Read the model definition and answer for the solid it produces. Units are mm, in the model's axes. Face numbers are marked on the shaded views. A direction names the side the tool comes from. Coordinates: 2 decimals unless noted, no trailing zeros. Write each loop counter-clockwise with the first axis right and the second up, starting at its lowest first coordinate (ties: lowest second). Pieces come first, ordered by that corner, then holes.
Item 1: A tool of negligible diameter and unlimited length cuts with its end or side. For the marked faces 1 and 2, from which of +Z, -Z, +X, -X, +Y, -Y can it reach the whole face along a straight path? Write none if from no direction.
Item 2: Straight lines are drawn through the part: probe 1 along X at (y, z) = (0, 12); probe 2 along X at (y, z) = (0, 1.2); probe 3 along Y at (x, z) = (32, 3). For each, find the intervals that lie inside material, in ascending order.
Item 3: Each of these flat-tipped pins is pushed along its axis until it touches: P1, Ø6, axis at x = -32, y = 0, coming from the +Z side; P2, Ø5, axis at x = -9.5, y = -26, coming from the -Z side; P3, Ø10, axis at x = 31, y = 2, coming from the +Z side. Where does it stop, or does it pass through?
Item 4: Section D-D (z = 31) is taken. Give the vertices of the cut face in (x, y), then the cut area to 3 significant figures.
Item 5: Section A-A (x = -2) is taken. Give the vertices of the cut face in (y, z), then the cut area to 3 significant figures.
Item 6: Section B-B (x = -32) is taken. Give the vertices of the cut face in (y, z), then the cut area to 3 significant figures.
Item 7: Section C-C (y = -16.5) is taken. Give the vertices of the cut face in (x, z).
from build123d import *

# Parameters (mm, degrees)
SKETCH1_W                = 80
SKETCH1_H                = 20
BOSS_EXTRUDE1_DEPTH      = 5
BOSS_EXTRUDE2_DEPTH      = 90
BOSS_EXTRUDE2_DEPTH_BACK = 64
SKETCH4_W                = 114
SKETCH4_H                = 22
CUT_EXTRUDE2_DEPTH       = 109.466361883
CHAMFER2_SIZE            = 11.3
CHAMFER2_SIZE_2          = 15.980613255
CHAMFER4_SIZE            = 5
CHAMFER4_SIZE2           = 10.722534603
CUT_EXTRUDE1_DEPTH       = 109.942423601
CUT_EXTRUDE1_DEPTH_BACK  = 109.942423601
SKETCH2_R                = 2.3
SKETCH5_R                = 4.5
CUT_EXTRUDE3_DEPTH       = 107.728174912
SKETCH6_R                = 1.5
CUT_EXTRUDE4_DEPTH       = 5
FILLET2_R                = 5.6


with BuildPart() as part:
    # Sketch1 → Boss-Extrude1 (new body)
    with BuildSketch(Plane.XY):
        Rectangle(SKETCH1_W, SKETCH1_H)
    extrude(amount=BOSS_EXTRUDE1_DEPTH)

    # Sketch3 → Boss-Extrude2 (add, two sides: drawn at the far end of the back side and taken through both)
    with BuildSketch(Plane(origin=(0, 0, 0), x_dir=(0, 0, -1), z_dir=(1, 0, 0)).offset(-BOSS_EXTRUDE2_DEPTH_BACK)):
        Polygon((-5, 10), (-50.254833996, -35.254833996), (-46.012193309, -35.254833996), (-5, 5.757359313), align=None)
    extrude(amount=BOSS_EXTRUDE2_DEPTH + BOSS_EXTRUDE2_DEPTH_BACK)

    # Sketch4 → Cut-Extrude2 (cut, through all)
    with BuildSketch(Plane(origin=(0, 5.378679656, 5.378679656), x_dir=(1, 0, 0), z_dir=(0, -0.7071067811865509, -0.7071067811865441))):
        with Locations((13, 33.464466094)):
            Rectangle(SKETCH4_W, SKETCH4_H)
    extrude(amount=-CUT_EXTRUDE2_DEPTH, mode=Mode.SUBTRACT)

    # Chamfer1
    # the kernel refuses this chamfer: 5 mm, written as the material it adds along each edge
    with BuildSketch(Plane(origin=(40, -25.102836543, 5), x_dir=(-0.027495876610586317, 0, -0.9996219169112968), z_dir=(0, 1, 0))) as chamfer1_piece_1_section:
        with BuildLine():
            Line((5.143365976, 0), (-0.282735774, -5.135588968))
            Line((-0.282735774, -5.135588968), (-0.382697966, -5.13283938))
            ThreePointArc((-0.382697966, -5.13283938), (-0.170646135, -2.566989148), (-0.099962192, 0.002749588))
            Line((-0.099962192, 0.002749588), (0.002749588, 0.099962192))
            ThreePointArc((0.002749588, 0.099962192), (2.572488324, 0.029278248), (5.146115564, 0.099962192))
            Line((5.146115564, 0.099962192), (5.143365976, 0))
        make_face()
    chamfer1_piece_1 = extrude(amount=35.102836543, mode=Mode.PRIVATE)
    chamfer1_piece_1 = split(chamfer1_piece_1, bisect_by=Plane(origin=(41.544288895, -10, 3.190389103), z_dir=(0, 1, 0)), keep=Keep.TOP, mode=Mode.PRIVATE)
    chamfer1_piece_1 = split(chamfer1_piece_1, bisect_by=Plane(origin=(41.544288895, -1.222319508, 0), z_dir=(0, 0, 1)), keep=Keep.TOP, mode=Mode.PRIVATE)
    chamfer1_piece_1 = split(chamfer1_piece_1, bisect_by=Plane(origin=(41.544288895, -1.222319508, 5), z_dir=(0, 0, -1)), keep=Keep.TOP, mode=Mode.PRIVATE)
    chamfer1_piece_1 = split(chamfer1_piece_1, bisect_by=Plane(origin=(41.544288895, 3.172325351, 7.585033962), z_dir=(0, -0.7071067811865511, -0.707106781186544)), keep=Keep.TOP, mode=Mode.PRIVATE)
    add(chamfer1_piece_1)
    with BuildSketch(Plane(origin=(40, -25.102836543, 5), x_dir=(-0.027495876610586317, 0, -0.9996219169112968), z_dir=(0, 1, 0))) as chamfer1_piece_2_section:
        with BuildLine():
            Line((5.143365976, 0), (-0.282735774, -5.135588968))
            Line((-0.282735774, -5.135588968), (-0.382697966, -5.13283938))
            ThreePointArc((-0.382697966, -5.13283938), (-0.170646135, -2.566989148), (-0.099962192, 0.002749588))
            Line((-0.099962192, 0.002749588), (0.002749588, 0.099962192))
            ThreePointArc((0.002749588, 0.099962192), (2.572488324, 0.029278248), (5.146115564, 0.099962192))
            Line((5.146115564, 0.099962192), (5.143365976, 0))
        make_face()
    chamfer1_piece_2 = extrude(amount=35.102836543, mode=Mode.PRIVATE)
    chamfer1_piece_2 = split(chamfer1_piece_2, bisect_by=Plane(origin=(41.882166071, 8.451075781, 5), z_dir=(0, 0, -1)), keep=Keep.TOP, mode=Mode.PRIVATE)
    chamfer1_piece_2 = split(chamfer1_piece_2, bisect_by=Plane(origin=(41.882166071, 7.676613671, 3.080745642), z_dir=(0, 0.7071067811865511, 0.707106781186544)), keep=Keep.TOP, mode=Mode.PRIVATE)
    add(chamfer1_piece_2)
    with BuildSketch(Plane(origin=(40, -25.102836543, 5), x_dir=(-0.027495876610586317, 0, -0.9996219169112968), z_dir=(0, 1, 0))) as chamfer1_piece_3_section:
        with BuildLine():
            Line((5.143365976, 0), (-0.282735774, -5.135588968))
            Line((-0.282735774, -5.135588968), (-0.382697966, -5.13283938))
            ThreePointArc((-0.382697966, -5.13283938), (-0.170646135, -2.566989148), (-0.099962192, 0.002749588))
            Line((-0.099962192, 0.002749588), (0.002749588, 0.099962192))
            ThreePointArc((0.002749588, 0.099962192), (2.572488324, 0.029278248), (5.146115564, 0.099962192))
            Line((5.146115564, 0.099962192), (5.143365976, 0))
        make_face()
    chamfer1_piece_3 = extrude(amount=35.102836543, mode=Mode.PRIVATE)
    chamfer1_piece_3 = split(chamfer1_piece_3, bisect_by=Plane(origin=(43.003980886, 7.808289703, 5), z_dir=(0, 0, 1)), keep=Keep.TOP, mode=Mode.PRIVATE)
    chamfer1_piece_3 = split(chamfer1_piece_3, bisect_by=Plane(origin=(43.003980886, 6.747629531, 4.009729782), z_dir=(0, 0.7071067811865511, 0.707106781186544)), keep=Keep.TOP, mode=Mode.PRIVATE)
    chamfer1_piece_3 = split(chamfer1_piece_3, bisect_by=Plane(origin=(43.003980886, 8.868949875, 6.131050125), z_dir=(0, -0.7071067811865511, -0.7071067811865439)), keep=Keep.TOP, mode=Mode.PRIVATE)
    add(chamfer1_piece_3)
    with BuildSketch(Plane(origin=(-40, 10, 5), x_dir=(0.027495876610586317, 0, -0.9996219169112968), z_dir=(0, -1, 0))) as chamfer1_piece_4_section:
        with BuildLine():
            Line((5.143365976, 0), (-0.282735774, -5.135588968))
            Line((-0.282735774, -5.135588968), (-0.382697966, -5.13283938))
            ThreePointArc((-0.382697966, -5.13283938), (-0.170646135, -2.566989148), (-0.099962192, 0.002749588))
            Line((-0.099962192, 0.002749588), (0.002749588, 0.099962192))
            ThreePointArc((0.002749588, 0.099962192), (2.572488324, 0.029278248), (5.146115564, 0.099962192))
            Line((5.146115564, 0.099962192), (5.143365976, 0))
        make_face()
    chamfer1_piece_4 = extrude(amount=35.102836543, mode=Mode.PRIVATE)
    chamfer1_piece_4 = split(chamfer1_piece_4, bisect_by=Plane(origin=(-41.882166071, 8.451075781, 5), z_dir=(0, 0, -1)), keep=Keep.TOP, mode=Mode.PRIVATE)
    chamfer1_piece_4 = split(chamfer1_piece_4, bisect_by=Plane(origin=(-41.882166071, 7.676613671, 3.080745642), z_dir=(0, 0.7071067811865511, 0.707106781186544)), keep=Keep.TOP, mode=Mode.PRIVATE)
    add(chamfer1_piece_4)
    with BuildSketch(Plane(origin=(-40, 10, 5), x_dir=(0.027495876610586317, 0, -0.9996219169112968), z_dir=(0, -1, 0))) as chamfer1_piece_5_section:
        with BuildLine():
            Line((5.143365976, 0), (-0.282735774, -5.135588968))
            Line((-0.282735774, -5.135588968), (-0.382697966, -5.13283938))
            ThreePointArc((-0.382697966, -5.13283938), (-0.170646135, -2.566989148), (-0.099962192, 0.002749588))
            Line((-0.099962192, 0.002749588), (0.002749588, 0.099962192))
            ThreePointArc((0.002749588, 0.099962192), (2.572488324, 0.029278248), (5.146115564, 0.099962192))
            Line((5.146115564, 0.099962192), (5.143365976, 0))
        make_face()
    chamfer1_piece_5 = extrude(amount=35.102836543, mode=Mode.PRIVATE)
    chamfer1_piece_5 = split(chamfer1_piece_5, bisect_by=Plane(origin=(-43.003980886, 7.808289703, 5), z_dir=(0, 0, 1)), keep=Keep.TOP, mode=Mode.PRIVATE)
    chamfer1_piece_5 = split(chamfer1_piece_5, bisect_by=Plane(origin=(-43.003980886, 6.747629531, 4.009729782), z_dir=(0, 0.7071067811865511, 0.707106781186544)), keep=Keep.TOP, mode=Mode.PRIVATE)
    chamfer1_piece_5 = split(chamfer1_piece_5, bisect_by=Plane(origin=(-43.003980886, 8.868949875, 6.131050125), z_dir=(0, -0.7071067811865511, -0.7071067811865439)), keep=Keep.TOP, mode=Mode.PRIVATE)
    add(chamfer1_piece_5)
    with BuildSketch(Plane(origin=(-40, 10, 5), x_dir=(0.027495876610586317, 0, -0.9996219169112968), z_dir=(0, -1, 0))) as chamfer1_piece_6_section:
        with BuildLine():
            Line((5.143365976, 0), (-0.282735774, -5.135588968))
            Line((-0.282735774, -5.135588968), (-0.382697966, -5.13283938))
            ThreePointArc((-0.382697966, -5.13283938), (-0.170646135, -2.566989148), (-0.099962192, 0.002749588))
            Line((-0.099962192, 0.002749588), (0.002749588, 0.099962192))
            ThreePointArc((0.002749588, 0.099962192), (2.572488324, 0.029278248), (5.146115564, 0.099962192))
            Line((5.146115564, 0.099962192), (5.143365976, 0))
        make_face()
    chamfer1_piece_6 = extrude(amount=35.102836543, mode=Mode.PRIVATE)
    chamfer1_piece_6 = split(chamfer1_piece_6, bisect_by=Plane(origin=(-41.544288895, -10, 3.190389103), z_dir=(0, 1, 0)), keep=Keep.TOP, mode=Mode.PRIVATE)
    chamfer1_piece_6 = split(chamfer1_piece_6, bisect_by=Plane(origin=(-41.544288895, -1.222319508, 0), z_dir=(0, 0, 1)), keep=Keep.TOP, mode=Mode.PRIVATE)
    chamfer1_piece_6 = split(chamfer1_piece_6, bisect_by=Plane(origin=(-41.544288895, -1.222319508, 5), z_dir=(0, 0, -1)), keep=Keep.TOP, mode=Mode.PRIVATE)
    chamfer1_piece_6 = split(chamfer1_piece_6, bisect_by=Plane(origin=(-41.544288895, 3.172325351, 7.585033962), z_dir=(0, -0.7071067811865511, -0.707106781186544)), keep=Keep.TOP, mode=Mode.PRIVATE)
    add(chamfer1_piece_6)

    # Chamfer2
    # the kernel refuses this chamfer: 15.980613255, 11.3 mm, written as the material it adds along each edge
    with BuildSketch(Plane(origin=(86.097071245, 5.757359313, 5), x_dir=(0, -0.6660419652145876, 0.745914271597675), z_dir=(-1, 0, 0))) as chamfer2_piece_1_section:
        Polygon((CHAMFER2_SIZE * 0.998403829789, -CHAMFER2_SIZE * 0.0564782494725), (CHAMFER2_SIZE_2 * 0.666041965207, -CHAMFER2_SIZE_2 * 0.745914271589), (0, 0), align=None)
    chamfer2_piece_1 = extrude(amount=172.194142489, mode=Mode.PRIVATE)
    chamfer2_piece_1 = split(chamfer2_piece_1, bisect_by=Plane(origin=(-23.869417759, -2.230051689, -16.130582241), z_dir=(0.7071067811862721, 0, 0.707106781186823)), keep=Keep.TOP, mode=Mode.PRIVATE)
    chamfer2_piece_1 = split(chamfer2_piece_1, bisect_by=Plane(origin=(23.869417759, -2.230051689, -16.130582241), z_dir=(-0.7071067811862721, 0, 0.707106781186823)), keep=Keep.TOP, mode=Mode.PRIVATE)
    chamfer2_piece_1 = split(chamfer2_piece_1, bisect_by=Plane(origin=(0, -10, 7.738835518), z_dir=(0, 1, 0)), keep=Keep.TOP, mode=Mode.PRIVATE)
    add(chamfer2_piece_1)

    # Chamfer4
    chamfer4_edges = [part.edges().sort_by_distance(p)[0] for p in [
        (0, -2.232947315, 12.990306627),
    ]]
    chamfer4_side = [part.faces().sort_by_distance(p)[0] for p in [
        (0, -6.014099628, 9.209154314),
    ]]
    chamfer(chamfer4_edges, length=CHAMFER4_SIZE, length2=CHAMFER4_SIZE2, reference=chamfer4_side[0])

    # Sketch2 → Cut-Extrude1 (cut, two sides: drawn at the far end of the back side and taken through both)
    with BuildSketch(Plane.XY.offset(-CUT_EXTRUDE1_DEPTH_BACK)):
        with Locations(Location((-32, 0, 0), (0, 0, 270))):
            Circle(SKETCH2_R)
        with Locations(Location((32, 0, 0), (0, 0, 270))):
            Circle(SKETCH2_R)
    extrude(amount=CUT_EXTRUDE1_DEPTH + CUT_EXTRUDE1_DEPTH_BACK, mode=Mode.SUBTRACT)

    # Sketch5 → Cut-Extrude3 (cut, through all)
    with BuildSketch(Plane(origin=(0, 0, 5), x_dir=(-1, 0, 0), z_dir=(0, 0, -1))):
        with Locations((-32, 0)):
            Circle(SKETCH5_R)
        with Locations((32, 0)):
            Circle(SKETCH5_R)
    extrude(amount=-CUT_EXTRUDE3_DEPTH, mode=Mode.SUBTRACT)

    # Sketch6 → Cut-Extrude4 (cut)
    with BuildSketch(Plane(origin=(0, 7.5, 7.5), x_dir=(1, 0, 0), z_dir=(0, 0.7071067811865511, 0.707106781186544))):
        with Locations(Location((-59.55, -4.214466094, 0), (0, 0, 270))):
            Circle(SKETCH6_R)
        with Locations(Location((-59.55, -53.714466094, 0), (0, 0, 270))):
            Circle(SKETCH6_R)
        with Locations(Location((84.95, -53.714466094, 0), (0, 0, 270))):
            Circle(SKETCH6_R)
        with Locations(Location((84.95, -4.214466094, 0), (0, 0, 270))):
            Circle(SKETCH6_R)
    extrude(amount=-CUT_EXTRUDE4_DEPTH, mode=Mode.SUBTRACT)

    # Fillet2
    fillet2_edges = [part.edges().sort_by_distance(p)[0] for p in [
        (-44, -9.445436483, 22.324116139),
        (-44, -25.001785669, 37.880465325),
        (70, -25.001785669, 37.880465325),
        (70, -9.445436483, 22.324116139),
    ]]
    fillet(fillet2_edges, radius=FILLET2_R)


solid = part.part
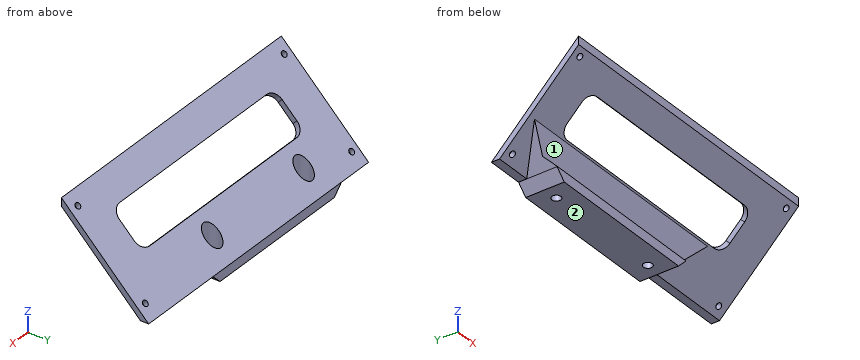
Established:
1. face 1: +X, -X, -Y
1. face 2: -Z, +X, -X, +Y, -Y
2. probe 1: x = -64 to -36.5, -27.5 to 27.5, 36.5 to 90
2. probe 2: x = -41.2 to -34.3, -29.7 to 29.7, 34.3 to 41.2
2. probe 3: y = -10 to -2.3, 2.3 to 10
3. P1: stops at z = 5
3. P2: stops at z = 36.82
3. P3: stops at z = 16.96
4. outline: (-64, -20.24) - (-44, -20.24) - (-44, -16) - (-64, -16) - close; (70, -20.24) - (90, -20.24) - (90, -16) - (70, -16) - close
4. area: 170 mm2
5. outline: (-35.25, 46.01) - (-26.06, 36.82) - (-23.94, 38.94) - (-35.25, 50.25) - close; (-10.51, 21.26) - (-9.81, 20.57) - (-5.77, 9.45) - (-10, 5.22) - (-10, 0) - (10, 0) - (10, 5) - (-8.38, 23.38) - close
5. area: 308 mm2
6. outline: (-35.25, 46.01) - (-26.06, 36.82) - (-23.94, 38.94) - (-35.25, 50.25) - close; (-10.51, 21.26) - (-9.81, 20.57) - (-5.77, 9.45) - (-10, 5.22) - (-10, 0) - (-2.3, 0) - (-2.3, 5) - (-4.5, 5) - (-4.5, 19.5) - (-8.38, 23.38) - close; (2.3, 0) - (10, 0) - (10, 5) - (4.5, 10.5) - (4.5, 5) - (2.3, 5) - close
6. area: 195 mm2
7. outline: (-64, 27.26) - (-44, 27.26) - (-44, 31.5) - (-64, 31.5) - close; (70, 27.26) - (90, 27.26) - (90, 31.5) - (70, 31.5) - close
